Work out the finished part from the listing and answer in its coordinate system (mm). Coordinates: 2 decimals unless noted, no trailing zeros. Order: outer loops, then holes, each group sorted by start corner. A loop starts at its lowest first (then second) coordinate and runs counter-clockwise, first axis right, second up. Notation, with made-up numbers: (66, 28) - (93, 28) arc R34 ccw to (93, 62) - close; hole circle Ø11 at (23, 41.25). An arc over 180 degrees is marked (long way). Answer as a JSON object with one key per item and string values. Group by question number.
1) Section C-C (x = -20) is taken. Give the vertices of the cut face in (y, z), plus the area to 3 significant figures.
2) Find the intervals of material crossed by line 1 along Y through (x, z) = (17.5, 9); line 2 along Z through (x, y) = (-24.5, 29); line 3 along Y through (x, z) = (6.5, 12), in increasing order.
3) Each of these flat-tipped pins is pushed along its axis until it touches: P1, Ø8, axis at x = -12.5, z = 14.5, coming from the -Y side; P2, Ø2, axis at y = 24, z = 16.5, coming from the +X side; P3, Ø12, axis at y = -5, z = 25, coming from the +X side; P4, Ø1.5, axis at x = 31.5, z = 16.5, coming from the -Y side. Where does it stop, or does it pass through?
4) Section A-A (y = 0) is taken. Give the vertices of the cut face in (x, z).
5) Section D-D (y = -23) is taken. Give the vertices of the cut face in (x, z), plus the area to 3 significant figures.
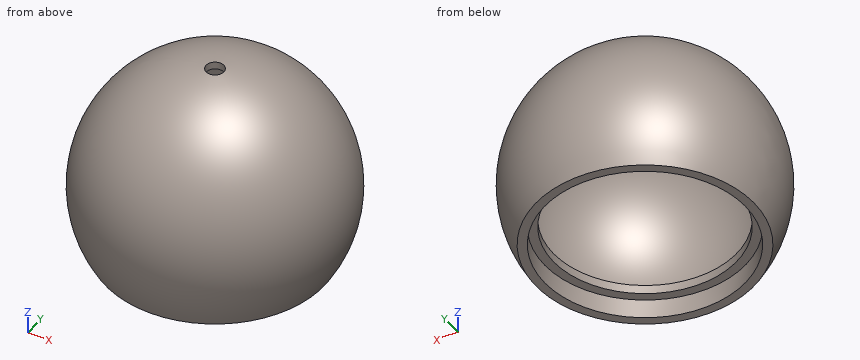
from build123d import *

# Parameters (mm, degrees)
F2_T      = -2.5
F3_R      = 34
F4_DEPTH  = 4.2
F6_R      = 3
F7_DEPTH  = 14
F8_R      = 36
F8_R_2    = 34
F9_DEPTH  = 4
F10_R     = 36
F10_R_2   = 31
F11_DEPTH = 3


with BuildPart() as f1:
    # F0 (on Front) → F1 (revolve)
    with BuildSketch(Plane.XZ):
        with BuildLine():
            Line((0, 0), (0, 65))
            ThreePointArc((0, 65), (-37.383151285, 43.2485293609), (-36.9459064038, 0))
            Line((-36.9459064038, 0), (0, 0))
        make_face()
    revolve(axis=Axis((0, 0, 20.3252808475), (0, 0, 1)))

    # F2 (hollow: no face is removed)
    offset(amount=F2_T, mode=Mode.SUBTRACT)

    # F3 (on face) → F4 (cut)
    with BuildSketch(Plane(origin=(0, 0, 0), x_dir=(1, 0, 0), z_dir=(0, 0, -1))):
        Circle(F3_R)
    extrude(amount=-F4_DEPTH, mode=Mode.SUBTRACT)

    # F6 (on offset) → F7 (cut)
    with BuildSketch(Plane.XY.offset(52)):
        Circle(F6_R)
    extrude(amount=F7_DEPTH, mode=Mode.SUBTRACT)

    # F8 (on face) → F9 (join)
    with BuildSketch(Plane.XY.offset(2.5)):
        Circle(F8_R)
        Circle(F8_R_2, mode=Mode.SUBTRACT)
    extrude(amount=F9_DEPTH)

    # F10 (on face) → F11 (join)
    with BuildSketch(Plane.XY.offset(6.5)):
        Circle(F10_R)
        Circle(F10_R_2, mode=Mode.SUBTRACT)
    extrude(amount=F11_DEPTH)


solid = f1.part
Report:
{
 "1": {"outline": "(-31.06, 0) - (-27.5, 0) - (-27.5, 6.5) - (-23.69, 6.5) - (-23.69, 9.5) - (-29.93, 9.5) - (-29.93, 3.45) arc R35.22 cw (long way) to (29.93, 3.45) - (29.93, 9.5) - (23.69, 9.5) - (23.69, 6.5) - (27.5, 6.5) - (27.5, 0) - (31.06, 0) arc R38.07 ccw (long way) to start", "area": "524 mm²"},
 "2": {"line 1": "y = -37.06 to -34.13, -31.46 to -25.59, 25.59 to 31.46, 34.13 to 37.06", "line 2": "z = 1.81 to 7.89, 36.11 to 42.19", "line 3": "y = -41.31 to -38.7, 38.7 to 41.31"},
 "3": {"P1": "stops at y = -41.68", "P2": "stops at x = 35.93", "P3": "stops at x = 43", "P4": "stops at y = -29.56"},
 "4": {"outline": "(-36.95, 0) - (-34, 0) - (-34, 6.5) - (-31, 6.5) - (-31, 9.5) - (-36, 9.5) - (-36, 3.45) arc R40.5 cw to (-3, 62.39) - (-3, 64.9) arc R43 ccw to start; (3, 62.39) arc R40.5 cw to (36, 3.45) - (36, 9.5) - (31, 9.5) - (31, 6.5) - (34, 6.5) - (34, 0) - (36.95, 0) arc R43 ccw to (3, 64.9) - close"},
 "5": {"outline": "(-28.91, 0) - (-25.04, 0) - (-25.04, 6.5) - (-20.78, 6.5) - (-20.78, 9.5) - (-27.69, 9.5) - (-27.69, 3.45) arc R33.34 cw (long way) to (27.69, 3.45) - (27.69, 9.5) - (20.78, 9.5) - (20.78, 6.5) - (25.04, 6.5) - (25.04, 0) - (28.91, 0) arc R36.33 ccw (long way) to start", "area": "538 mm²"}
}
